Here's how the part is built. I have some questions about the finished solid (model axes, mm). Face numbers are marked on the shaded views. A direction names the side the tool comes from. Coordinates: 2 decimals unless noted, no trailing zeros. Write each loop counter-clockwise with the first axis right and the second up, starting at its lowest first coordinate (ties: lowest second). Pieces come first, ordered by that corner, then holes. Notation, with made-up numbers: (6, 85) -> (59, 85) arc R22 ccw to (59, 105) -> close; hole circle Ø10 at (-16, 61.25). An arc over 180 degrees is marked (long way). Put each result on its own line as item: value. Start each with the question number.
Item 1: I want a section at C-C, the plane x = -3.25. List the corners of the cut face in (y, z) for me.
Item 2: I need wall thicknesses on line 1 (X direction, y = -11, z = 8.25); line 2 (Y direction, x = 12.5, z = 1.25); line 3 (X direction, y = 10.5, z = 14.25). Which ranges of each line are inside material? Lowest first, please. Write a range as [from, to].
Item 3: For pin 1 (2.5 mm diameter, centred on x = 12, z = 14.5, fed in from -Y); pin 2 (1.5 mm diameter, centred on y = -12.5, z = 14, fed in from +X); pin 3 (10 mm diameter, centred on x = -5.5, z = 10.5, fed in from -Y), each with a flat end and sliding along its axis, tell me the tip position at first contact or that it passes through.
Item 4: I want a section at A-A, the plane z = 8.5. List the corners of the cut face in (x, y) for me, then the cut area to 3 significant figures.
Item 5: I want a section at B-B, the plane y = -7.5. List the corners of the cut face in (x, z) for me, then the cut area to 3 significant figures.
Item 6: On a 3-axis mill with a long thin cutter (end or side, diameter ignored), from which of +Z, -Z, +X, -X, +Y, -Y can I reach the whole of each face in a straight line? I mean the marked faces 1 and 2. Say none if no direction works.
from build123d import *

# Parameters (mm, degrees)
EXTRUDE_1_DEPTH = 20


with BuildPart() as part:
    # 草圖1 → 填料-伸長1 (new body)
    with BuildSketch(Plane.XY):
        Polygon((-11, -11), (11, 11), (14, 11), (14, 14), (-14, 14), (-14, -14), (-11, -14), align=None)
    extrude(amount=EXTRUDE_1_DEPTH)


solid = part.part
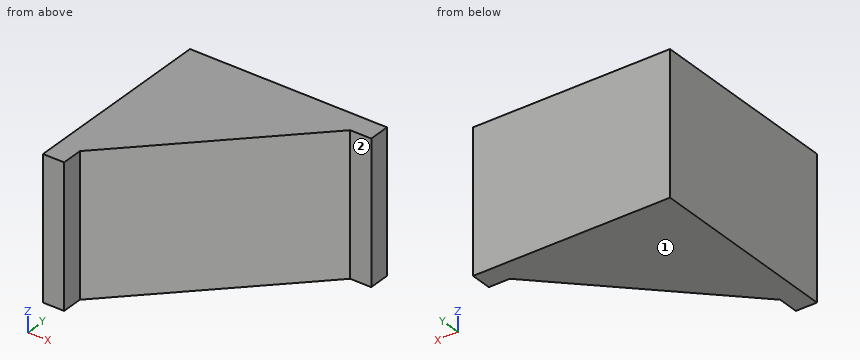
Calculated:
1. outline: (-3.25, 0) -> (14, 0) -> (14, 20) -> (-3.25, 20) -> close
2. line 1: x = [-14, -11]
2. line 2: y = [11, 14]
2. line 3: x = [-14, 10.5]
3. pin 1: stops at y = 10.75
3. pin 2: stops at x = -11
3. pin 3: stops at y = -10.5
4. outline: (-14, -14) -> (-11, -14) -> (-11, -11) -> (11, 11) -> (14, 11) -> (14, 14) -> (-14, 14) -> close
4. area: 401 mm2
5. outline: (-14, 0) -> (-7.5, 0) -> (-7.5, 20) -> (-14, 20) -> close
5. area: 130 mm2
6. face 1: -Z, +X, -X, +Y, -Y
6. face 2: +Z, -Z, +X, -Y
